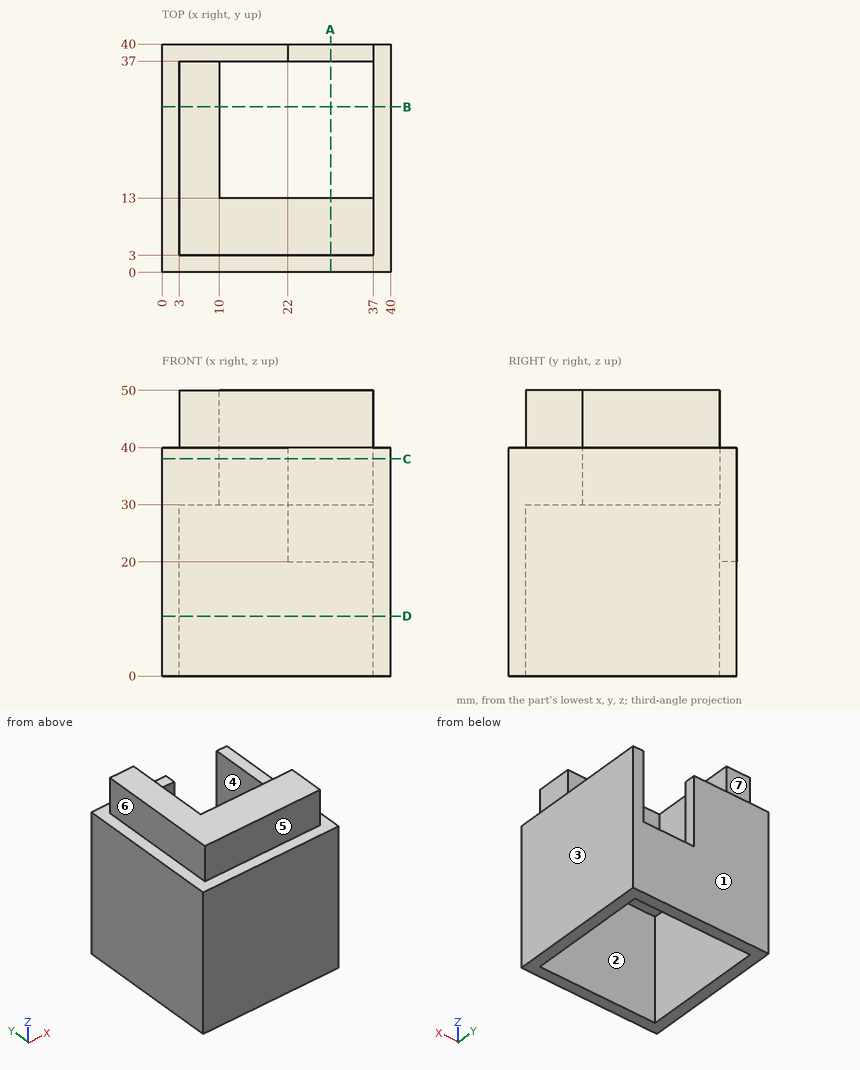
Geometry: see drawing. Coordinates: mm, zero at the bounding-box minimum. A direction names the side the tool comes from. Round coordinates to 2 decimals unless told otherwise and drop trailing zeros. Order: outer loops, then holes, each group sorted by start corner. A loop starts at its lowest first (then second) coordinate and runs counter-clockwise, first axis right, second up. Notation, with made-up numbers: (55.5, 2) - (61.5, 2) arc R31 cw to (61.5, 38) - close; hole circle Ø8 at (-11.75, -14). An arc over 180 degrees is marked (long way). One line per question, with ' | ' between items. Start each with the question number.
1) Set-up query: the marked faces 5, 6 and 7. Return all of +Z, -Z, +X, -X, +Y, -Y with unobstructed straight access to the full face (end or side cutting, diameter ignored); none if empty.
2) Cut plane C-C, the plane z = 38. Return the cut outline in (x, y), then the cut area to 3 significant figures.
3) Cut plane D-D, the plane z = 10.5. Return the cut outline in (x, y).
4) Ray query, probe 1 along X at (y, z) = (22, 37); probe 2 along X at (y, z) = (16, 4). Return the intervals inside material, ascending.
5) Cut plane B-B, the plane y = 29. Return the cut outline in (x, z).
6) Cut plane A-A, the plane x = 29.5. Return the cut outline in (y, z).
7) Pull-direction query (Y, two-part tool) for the marked faces 1, 2, 3 and 4; classes: +Y half, -Y half, draft (parallel to the pull), parting line (faces both ways), or undercut.
8) Contact query for flat-ended pins moving along their axis: P1, Ø0.9, axis at x = 26, y = 39, coming from the +Z side; P2, Ø3.5, axis at x = 5.5, z = 46.5, coming from the +Y side; P3, Ø5, axis at y = 6.5, z = 43, coming from the +X side. Output: stop coordinate, or through.
Worked out:
1) face 5: +Z, +X, -X, -Y | face 6: +Z, -X, +Y, -Y | face 7: +Z, +X, -X, +Y
2) outline: (0, 0) - (40, 0) - (40, 40) - (37, 40) - (37, 13) - (10, 13) - (10, 37) - (22, 37) - (22, 40) - (0, 40) - close | area: 907 mm^2
3) outline: (0, 0) - (40, 0) - (40, 40) - (0, 40) - close; hole (3, 3) - (37, 3) - (37, 37) - (3, 37) - close
4) probe 1: x = 0 to 10, 37 to 40 | probe 2: x = 0 to 3, 37 to 40
5) outline: (0, 0) - (3, 0) - (3, 30) - (10, 30) - (10, 50) - (3, 50) - (3, 40) - (0, 40) - close; (37, 0) - (40, 0) - (40, 40) - (37, 40) - close
6) outline: (0, 0) - (3, 0) - (3, 30) - (13, 30) - (13, 50) - (3, 50) - (3, 40) - (0, 40) - close; (37, 0) - (40, 0) - (40, 20) - (37, 20) - close
7) face 1: +Y half | face 2: undercut | face 3: draft | face 4: undercut
8) P1: stops at z = 20 | P2: stops at y = 37 | P3: stops at x = 37
